```python
from build123d import *

# Parameters (mm, degrees)
SKICA1_W                 = 23.7
SKICA1_H                 = 48.55
SKICA1_W_2               = 23
SKICA1_H_2               = 22
P_IDAT_VYSUNUT_M1_DEPTH  = 2
SKICA3_R                 = 3
ODEBRAT_VYSUNUT_M1_DEPTH = 4
ZKOSEN_1_SIZE            = 3.464101615
ZKOSEN_1_SIZE_2          = 2
SKICA5_W                 = 44
SKICA5_H                 = 108
SKICA5_W_2               = 40
SKICA5_H_2               = 104
P_IDAT_VYSUNUT_M3_DEPTH  = 6
ZAOBLIT2_R               = 2.5
SKICA6_W                 = 27
SKICA6_H                 = 26
SKICA6_W_2               = 23
SKICA6_H_2               = 22
P_IDAT_VYSUNUT_M4_DEPTH  = 7
SKICA7_R                 = 1
P_IDAT_VYSUNUT_M5_DEPTH  = 2
SKICA8_W                 = 23
SKICA8_H                 = 1
ODEBRAT_VYSUNUT_M3_DEPTH = 30
SKICA9_W                 = 1
SKICA9_H                 = 22
ODEBRAT_VYSUNUT_M4_DEPTH = 30
ZAOBLIT3_R               = 2
SKICA10_W                = 42
SKICA10_H                = 106
SKICA10_W_2              = 40
SKICA10_H_2              = 104
ODEBRAT_VYSUNUT_M5_DEPTH = 2


# Some blends are built 0.0001 mm under size
with BuildPart() as part:
    # Skica1 → Přidat vysunutím1 (new body)
    with BuildSketch(Plane.XY):
        Polygon((-10.15, 2), (-10.15, 25), (33.85, 25), (33.85, 2), (33.85, -83), (-10.15, -83), (-10.15, -61.55), align=None)
        with Locations((11.85, -37.275)):
            Rectangle(SKICA1_W, SKICA1_H, mode=Mode.SUBTRACT)
        with Locations((11.85, 9)):
            Rectangle(SKICA1_W_2, SKICA1_H_2, mode=Mode.SUBTRACT)
    extrude(amount=P_IDAT_VYSUNUT_M1_DEPTH)

    # Skica3 → Odebrat vysunutím1 (cut)
    with BuildSketch(Plane.XY.offset(2)):
        with Locations((11.85, -77.5)):
            Circle(SKICA3_R)
    extrude(amount=-ODEBRAT_VYSUNUT_M1_DEPTH, mode=Mode.SUBTRACT)

    # Zkosení1
    # the kernel refuses this chamfer: 3.464101615, 2 mm, written as the material it takes off along each edge
    with BuildSketch(Plane(origin=(0, -13, 0), x_dir=(-0.9998132206222079, 0, -0.019326765612700626), z_dir=(0, -1, 0)), Plane(origin=(23.7, -61.55, 0), x_dir=(0.9998132206222079, 0, -0.019326765612700608), z_dir=(0, 1, 0))) as zkosen_1_piece_1:
        Polygon((ZKOSEN_1_SIZE * 0.999813220662, -ZKOSEN_1_SIZE * 0.0193267656135), (-ZKOSEN_1_SIZE_2 * 0.0193267656127, -ZKOSEN_1_SIZE_2 * 0.999813220622), (0, 0), align=None)
    extrude(amount=48.55, mode=Mode.SUBTRACT)
    with BuildSketch(Plane(origin=(0, -61.55, 0), x_dir=(0, -0.9998132206222079, -0.01932676561270056), z_dir=(1, 0, 0)), Plane(origin=(23.7, -13, 0), x_dir=(0, 0.9998132206222079, -0.019326765612700643), z_dir=(-1, 0, 0))) as zkosen_1_piece_2:
        Polygon((ZKOSEN_1_SIZE * 0.999813220662, -ZKOSEN_1_SIZE * 0.0193267656135), (-ZKOSEN_1_SIZE_2 * 0.0193267656127, -ZKOSEN_1_SIZE_2 * 0.999813220622), (0, 0), align=None)
    extrude(amount=23.7, mode=Mode.SUBTRACT)
    with BuildSketch(Plane(origin=(0, -4.038072059, 0), x_dir=(-0.9998132206222079, 0, -0.019326765612700622), z_dir=(0, -1, 0))) as zkosen_1_piece_3a_section:
        Polygon((ZKOSEN_1_SIZE * 0.999813220662, -ZKOSEN_1_SIZE * 0.0193267656135), (-ZKOSEN_1_SIZE_2 * 0.0193267656127, -ZKOSEN_1_SIZE_2 * 0.999813220622), (0, 0), align=None)
    zkosen_1_piece_3a = extrude(amount=57.511927941, mode=Mode.PRIVATE)
    zkosen_1_piece_3a = split(zkosen_1_piece_3a, bisect_by=Plane(origin=(-1.161798269, -13, 0.64133979), z_dir=(0, 1, 0)), keep=Keep.TOP, mode=Mode.PRIVATE)
    with BuildSketch(Plane(origin=(23.7, -13, 0), x_dir=(0, 0.9998132206222079, -0.019326765612700643), z_dir=(-1, 0, 0))) as zkosen_1_piece_3b_section:
        Polygon((ZKOSEN_1_SIZE * 0.999813220662, -ZKOSEN_1_SIZE * 0.0193267656135), (-ZKOSEN_1_SIZE_2 * 0.0193267656127, -ZKOSEN_1_SIZE_2 * 0.999813220622), (0, 0), align=None)
    zkosen_1_piece_3b = extrude(amount=32.661927941, mode=Mode.PRIVATE)
    zkosen_1_piece_3b = split(zkosen_1_piece_3b, bisect_by=Plane(origin=(0, -11.838201731, 0.64133979), z_dir=(-1, 0, 0)), keep=Keep.TOP, mode=Mode.PRIVATE)
    zkosen_1_piece_3 = zkosen_1_piece_3a & zkosen_1_piece_3b
    add(zkosen_1_piece_3, mode=Mode.SUBTRACT)
    with BuildSketch(Plane(origin=(0, -13, 0), x_dir=(-0.9998132206222079, 0, -0.019326765612700626), z_dir=(0, -1, 0))) as zkosen_1_piece_4a_section:
        Polygon((ZKOSEN_1_SIZE * 0.999813220662, -ZKOSEN_1_SIZE * 0.0193267656135), (-ZKOSEN_1_SIZE_2 * 0.0193267656127, -ZKOSEN_1_SIZE_2 * 0.999813220622), (0, 0), align=None)
    zkosen_1_piece_4a = extrude(amount=57.511927941, mode=Mode.PRIVATE)
    zkosen_1_piece_4a = split(zkosen_1_piece_4a, bisect_by=Plane(origin=(-1.161798269, -61.55, 0.64133979), z_dir=(0, -1, 0)), keep=Keep.TOP, mode=Mode.PRIVATE)
    with BuildSketch(Plane(origin=(-8.961927941, -61.55, 0), x_dir=(0, -0.9998132206222079, -0.01932676561270056), z_dir=(1, 0, 0))) as zkosen_1_piece_4b_section:
        Polygon((ZKOSEN_1_SIZE * 0.999813220662, -ZKOSEN_1_SIZE * 0.0193267656135), (-ZKOSEN_1_SIZE_2 * 0.0193267656127, -ZKOSEN_1_SIZE_2 * 0.999813220622), (0, 0), align=None)
    zkosen_1_piece_4b = extrude(amount=32.661927941, mode=Mode.PRIVATE)
    zkosen_1_piece_4b = split(zkosen_1_piece_4b, bisect_by=Plane(origin=(0, -62.711798269, 0.64133979), z_dir=(-1, 0, 0)), keep=Keep.TOP, mode=Mode.PRIVATE)
    zkosen_1_piece_4 = zkosen_1_piece_4a & zkosen_1_piece_4b
    add(zkosen_1_piece_4, mode=Mode.SUBTRACT)
    with BuildSketch(Plane(origin=(0, -61.55, 0), x_dir=(0, -0.9998132206222079, -0.01932676561270056), z_dir=(1, 0, 0))) as zkosen_1_piece_5a_section:
        Polygon((ZKOSEN_1_SIZE * 0.999813220662, -ZKOSEN_1_SIZE * 0.0193267656135), (-ZKOSEN_1_SIZE_2 * 0.0193267656127, -ZKOSEN_1_SIZE_2 * 0.999813220622), (0, 0), align=None)
    zkosen_1_piece_5a = extrude(amount=32.661927941, mode=Mode.PRIVATE)
    zkosen_1_piece_5a = split(zkosen_1_piece_5a, bisect_by=Plane(origin=(23.7, -62.711798269, 0.64133979), z_dir=(1, 0, 0)), keep=Keep.TOP, mode=Mode.PRIVATE)
    with BuildSketch(Plane(origin=(23.7, -70.511927941, 0), x_dir=(0.9998132206222079, 0, -0.019326765612700608), z_dir=(0, 1, 0))) as zkosen_1_piece_5b_section:
        Polygon((ZKOSEN_1_SIZE * 0.999813220662, -ZKOSEN_1_SIZE * 0.0193267656135), (-ZKOSEN_1_SIZE_2 * 0.0193267656127, -ZKOSEN_1_SIZE_2 * 0.999813220622), (0, 0), align=None)
    zkosen_1_piece_5b = extrude(amount=57.511927941, mode=Mode.PRIVATE)
    zkosen_1_piece_5b = split(zkosen_1_piece_5b, bisect_by=Plane(origin=(24.861798269, -61.55, 0.64133979), z_dir=(0, -1, 0)), keep=Keep.TOP, mode=Mode.PRIVATE)
    zkosen_1_piece_5 = zkosen_1_piece_5a & zkosen_1_piece_5b
    add(zkosen_1_piece_5, mode=Mode.SUBTRACT)
    with BuildSketch(Plane(origin=(32.661927941, -13, 0), x_dir=(0, 0.9998132206222079, -0.019326765612700643), z_dir=(-1, 0, 0))) as zkosen_1_piece_6a_section:
        Polygon((ZKOSEN_1_SIZE * 0.999813220662, -ZKOSEN_1_SIZE * 0.0193267656135), (-ZKOSEN_1_SIZE_2 * 0.0193267656127, -ZKOSEN_1_SIZE_2 * 0.999813220622), (0, 0), align=None)
    zkosen_1_piece_6a = extrude(amount=32.661927941, mode=Mode.PRIVATE)
    zkosen_1_piece_6a = split(zkosen_1_piece_6a, bisect_by=Plane(origin=(23.7, -11.838201731, 0.64133979), z_dir=(1, 0, 0)), keep=Keep.TOP, mode=Mode.PRIVATE)
    with BuildSketch(Plane(origin=(23.7, -61.55, 0), x_dir=(0.9998132206222079, 0, -0.019326765612700608), z_dir=(0, 1, 0))) as zkosen_1_piece_6b_section:
        Polygon((ZKOSEN_1_SIZE * 0.999813220662, -ZKOSEN_1_SIZE * 0.0193267656135), (-ZKOSEN_1_SIZE_2 * 0.0193267656127, -ZKOSEN_1_SIZE_2 * 0.999813220622), (0, 0), align=None)
    zkosen_1_piece_6b = extrude(amount=57.511927941, mode=Mode.PRIVATE)
    zkosen_1_piece_6b = split(zkosen_1_piece_6b, bisect_by=Plane(origin=(24.861798269, -13, 0.64133979), z_dir=(0, 1, 0)), keep=Keep.TOP, mode=Mode.PRIVATE)
    zkosen_1_piece_6 = zkosen_1_piece_6a & zkosen_1_piece_6b
    add(zkosen_1_piece_6, mode=Mode.SUBTRACT)

    # Skica5 → Přidat vysunutím3 (add)
    with BuildSketch(Plane.XY.offset(2)):
        with Locations((11.85, -29)):
            Rectangle(SKICA5_W, SKICA5_H)
        with Locations((11.85, -29)):
            Rectangle(SKICA5_W_2, SKICA5_H_2, mode=Mode.SUBTRACT)
    extrude(amount=P_IDAT_VYSUNUT_M3_DEPTH)

    # Zaoblit2
    zaoblit2_edges = [part.edges().sort_by_distance(p)[0] for p in [
        (33.85, -83, 4),
        (-10.15, -83, 4),
        (-10.15, 25, 4),
        (33.85, 25, 4),
        (33.85, -29, 0),
        (11.85, -83, 0),
        (-10.15, -29, 0),
        (11.85, 25, 0),
    ]]
    fillet(zaoblit2_edges, radius=ZAOBLIT2_R - 0.0001)  # a hair under: the kernel refuses the full size

    # Skica6 → Přidat vysunutím4 (add)
    with BuildSketch(Plane(origin=(0, 0, 0), x_dir=(-1, 0, 0), z_dir=(0, 0, -1))):
        with Locations((-11.85, 9)):
            Rectangle(SKICA6_W, SKICA6_H)
        with Locations((-11.85, 9)):
            Rectangle(SKICA6_W_2, SKICA6_H_2, mode=Mode.SUBTRACT)
    extrude(amount=P_IDAT_VYSUNUT_M4_DEPTH)

    # Skica7 → Přidat vysunutím5 (add)
    # profile 1 of 4: a face of its own
    with BuildSketch(Plane(origin=(0, 0, 0), x_dir=(-1, 0, 0), z_dir=(0, 0, -1))):
        with BuildLine():
            Line((-23.35, -2), (-23.35, 4))
            ThreePointArc((-23.35, 4), (-19.107359313, 2.242640687), (-17.35, -2))
            Line((-17.35, -2), (-23.35, -2))
        make_face()
        with Locations((-20.85, 0.5)):
            Circle(SKICA7_R, mode=Mode.SUBTRACT)
    # profile 2 of 4: a face of its own
    with BuildSketch(Plane(origin=(0, 0, 0), x_dir=(-1, 0, 0), z_dir=(0, 0, -1))):
        with BuildLine():
            Line((-0.35, 20), (-6.35, 20))
            ThreePointArc((-6.35, 20), (-4.592640687, 15.757359313), (-0.35, 14))
            Line((-0.35, 14), (-0.35, 20))
        make_face()
        with Locations((-2.85, 17.5)):
            Circle(SKICA7_R, mode=Mode.SUBTRACT)
    # profile 3 of 4: a face of its own
    with BuildSketch(Plane(origin=(0, 0, 0), x_dir=(-1, 0, 0), z_dir=(0, 0, -1))):
        with BuildLine():
            Line((-0.35, -2), (-0.35, 4))
            ThreePointArc((-0.35, 4), (-4.592640687, 2.242640687), (-6.35, -2))
            Line((-6.35, -2), (-0.35, -2))
        make_face()
        with Locations((-2.85, 0.5)):
            Circle(SKICA7_R, mode=Mode.SUBTRACT)
    # profile 4 of 4: a face of its own
    with BuildSketch(Plane(origin=(0, 0, 0), x_dir=(-1, 0, 0), z_dir=(0, 0, -1))):
        with BuildLine():
            Line((-23.35, 20), (-23.35, 14))
            ThreePointArc((-23.35, 14), (-19.107359313, 15.757359313), (-17.35, 20))
            Line((-17.35, 20), (-23.35, 20))
        make_face()
        with Locations((-20.85, 17.5)):
            Circle(SKICA7_R, mode=Mode.SUBTRACT)
    extrude(amount=-P_IDAT_VYSUNUT_M5_DEPTH)

    # Skica8 → Odebrat vysunutím3 (cut)
    with BuildSketch(Plane.XZ.offset(4)):
        with Locations((11.85, -5.5)):
            Rectangle(SKICA8_W, SKICA8_H)
        with Locations((11.85, -3.5)):
            Rectangle(SKICA8_W, SKICA8_H)
        with Locations((11.85, -1.5)):
            Rectangle(SKICA8_W, SKICA8_H)
    extrude(amount=-ODEBRAT_VYSUNUT_M3_DEPTH, mode=Mode.SUBTRACT)

    # Skica9 → Odebrat vysunutím4 (cut)
    with BuildSketch(Plane.ZY.offset(1.65)):
        with Locations((-5.5, 9)):
            Rectangle(SKICA9_W, SKICA9_H)
        with Locations((-3.5, 9)):
            Rectangle(SKICA9_W, SKICA9_H)
        with Locations((-1.5, 9)):
            Rectangle(SKICA9_W, SKICA9_H)
    extrude(amount=-ODEBRAT_VYSUNUT_M4_DEPTH, mode=Mode.SUBTRACT)

    # Zaoblit3
    zaoblit3_edges = [part.edges().sort_by_distance(p)[0] for p in [
        (-1.65, -4, -3.5),
        (-1.65, 22, -3.5),
        (25.35, 22, -3.5),
        (25.35, -4, -3.5),
    ]]
    fillet(zaoblit3_edges, radius=ZAOBLIT3_R - 0.0001)  # a hair under: the kernel refuses the full size

    # Skica10 → Odebrat vysunutím5 (cut)
    with BuildSketch(Plane.XY.offset(8)):
        with Locations((11.85, -29)):
            Rectangle(SKICA10_W, SKICA10_H)
        with Locations((11.85, -29)):
            Rectangle(SKICA10_W_2, SKICA10_H_2, mode=Mode.SUBTRACT)
    extrude(amount=-ODEBRAT_VYSUNUT_M5_DEPTH, mode=Mode.SUBTRACT)


solid = part.part
```
Read the model definition and answer for the solid it produces. Units are mm, in the model's axes. A direction names the side the tool comes from. Coordinates: 2 decimals unless noted, no trailing zeros. Loops run counter-clockwise (first coordinate to the right, second up) from the corner with the lowest first, then second, coordinate; pieces in that order, holes last. Notation, with made-up numbers: (11, 1) - (39, 1) arc R14 cw to (39, 21) - close; hole circle Ø8 at (-5.75, -11.5). An arc over 180 degrees is marked (long way). Answer in a Markdown table with one row per item.
1. Which of the six approach directions +Z, -Z, +X, -X, +Y, -Y give full straight-line access (tool end or side, diameter ignored) to faces 4 (the face through (-8.15, -30, 4)), 5 (the face through (23.35, 9, 0)), 6 (the face through (12, -3, -6)), 7 (the face through (24.78, -3.4, -3.55))?
Conclusion:
| item | result |
|---|---|
| face 4 | +Z |
| face 5 | -Z |
| face 6 | +Y, -Y |
| face 7 | -Z, +X, -Y |
2. Determine the mould class of faces 1 (the face through (24, 9, -6)), 2 (the face through (4.546, 2.289, 0.986)), 3 (the face through (-9.437, -82.248, 5.288)) for opening direction X: +X half, -X half, draft (parallel to the pull), parting line (faces both ways), or undercut.
Conclusion:
| item | result |
|---|---|
| face 1 | draft |
| face 2 | undercut |
| face 3 | -X half |
3. Find section B-B, the plane x = 11.85. Count the separate pieces of the cut face and the enclosed holes in it, then the cut area to 3 significant figures.
Conclusion:
| item | result |
|---|---|
| separate pieces | 10 |
| enclosed holes | 0 |
| area | 89.3 mm² |
4. Find section D-D, the plane y = -77.5. Write down the section's boundary in (x, z), then the cut area to 3 significant figures.
Conclusion:
| item | result |
|---|---|
| outline | (-10.15, 2.5) arc R2.5 ccw to (-7.65, 0) - (8.85, 0) - (8.85, 2) - (-8.15, 2) - (-8.15, 6) - (-9.15, 6) - (-9.15, 8) - (-10.15, 8) - close; (14.85, 0) - (31.35, 0) arc R2.5 ccw to (33.85, 2.5) - (33.85, 8) - (32.85, 8) - (32.85, 6) - (31.85, 6) - (31.85, 2) - (14.85, 2) - close |
| area | 93.3 mm² |
5. Find section A-A, the plane y = -15. Write down the section's boundary in (x, z), then the cut area to 3 significant figures.
Conclusion:
| item | result |
|---|---|
| outline | (-10.15, 2.5) arc R2.5 ccw to (-7.65, 0) - (-3.46, 0) - (0, 2) - (-8.15, 2) - (-8.15, 6) - (-9.15, 6) - (-9.15, 8) - (-10.15, 8) - close; (23.7, 2) - (27.16, 0) - (31.35, 0) arc R2.5 ccw to (33.85, 2.5) - (33.85, 8) - (32.85, 8) - (32.85, 6) - (31.85, 6) - (31.85, 2) - close |
| area | 51.0 mm² |
6. Straight lines are drawn through the part: line 1 (Z direction, x = 20, y = -2.5); line 2 (Y direction, x = 23, z = 7); line 3 (Y direction, x = 4, z = 3). For each, find the intervals that lie inside material, in ascending order.
Conclusion:
| item | result |
|---|---|
| line 1 | z = -7 to -6, -5 to -4, -3 to -2, -1 to 2 |
| line 2 | y = -83 to -82, 24 to 25 |
| line 3 | y = -83 to -81, 23 to 25 |
7. Given pin 1 (2 mm diameter, centred on x = 29.5, y = -45, fed in from -Z); pin 2 (0.9 mm diameter, centred on x = 12.5, z = 0.5, fed in from -Y); pin 3 (0.8 mm diameter, centred on x = -0.5, z = -1.5, fed in from -Y), each flat-ended and moving along its own axis, determine where each tip first touches the part or whether it passes through.
Conclusion:
| item | result |
|---|---|
| pin 1 | stops at z = 0 |
| pin 2 | stops at y = -82.46 |
| pin 3 | stops at y = -3.95 |
